```python
from build123d import *

# Parameters (mm, degrees)
SKETCH1_W           = 299.7
SKETCH1_H           = 56.55
BOSS_EXTRUDE1_DEPTH = 3.175
SKETCH2_W           = 144
SKETCH2_H           = 3.175
BOSS_EXTRUDE2_DEPTH = 6.35


with BuildPart() as part:
    # Sketch1 → Boss-Extrude1 (new body)
    with BuildSketch(Plane.XY):
        Rectangle(SKETCH1_W, SKETCH1_H)
    extrude(amount=BOSS_EXTRUDE1_DEPTH)

    # Sketch2 → Boss-Extrude2 (add)
    with BuildSketch(Plane.XZ.offset(28.275)):
        with Locations((0, 1.5875)):
            Rectangle(SKETCH2_W, SKETCH2_H)
    extrude(amount=BOSS_EXTRUDE2_DEPTH)


solid = part.part
```
For this review, take the finished solid that the model builds, in its own axes (mm). Coordinates: 2 decimals unless noted, no trailing zeros. Write each loop counter-clockwise with the first axis right and the second up, starting at its lowest first coordinate (ties: lowest second). Pieces come first, ordered by that corner, then holes. Notation, with made-up numbers: (-30, -30) -> (-12, -30) arc R21 cw to (-12, -3) -> close; hole circle Ø11 at (27, 25.25). An arc over 180 degrees is marked (long way). Put each result on its own line as item: value.
Q1. Wall thickness on L1, parallel to Y at x = 119, z = 0.6 (3 decimals): over which ranges is the line inside the solid? List them lowest first.
From the geometry:
L1: y = -28.275 to 28.275
Q2. Take a section at B-B, the plane x = 99. State the section outline as (y, z) points (3 decimals).
From the geometry:
outline: (-28.275, 0) -> (28.275, 0) -> (28.275, 3.175) -> (-28.275, 3.175) -> close
Q3. Take a section at A-A, the plane z = 1.9. State the section outline as (x, y) points (3 decimals).
From the geometry:
outline: (-149.85, -28.275) -> (-72, -28.275) -> (-72, -34.625) -> (72, -34.625) -> (72, -28.275) -> (149.85, -28.275) -> (149.85, 28.275) -> (-149.85, 28.275) -> close
Q4. Clearance check with flat-ended pins moving along their axes: pin 1 Ø1 at (y, z) = (-32.5, 2) entering from -X; pin 2 Ø1.6 at (x, z) = (113.5, 1.5) entering from -Y (3 decimals); pin 3 Ø1 at (y, z) = (-30.5, 2) entering from +X. State where each tip first meets the part, or that it passes through.
From the geometry:
pin 1: stops at x = -72
pin 2: stops at y = -28.275
pin 3: stops at x = 72
